For this review, take the finished solid that the model builds, in its own axes (mm). Face numbers are marked on the shaded views. Round coordinates to 2 decimals unless told otherwise and drop trailing zeros. Write each loop counter-clockwise with the first axis right and the second up, starting at its lowest first coordinate (ties: lowest second). Pieces come first, ordered by that corner, then holes. Notation, with made-up numbers: (70, 38.25) - (79, 38.25) arc R18 ccw to (79, 42.25) - close; hole circle Ø10 at (-34, 38). An arc over 180 degrees is marked (long way). One line per item, written item: value. Start each with the question number.
Q1. Add section C-C on z = 38. Write out the cut boundary in (x, y) (1 decimal), and give its area (3 significant figures).
Q2. Clearance check with flat-ended pins moving along their axes: pin 1 Ø5 at (y, z) = (1.5, 21) entering from +X; pin 2 Ø3 at (y, z) = (-4.5, 26) entering from +X; pin 3 Ø5 at (x, z) = (6, 38) entering from +Y; pin 4 Ø1.5 at (y, z) = (2, 42) entering from -X. State where each tip first meets the part, or that it passes through.
Q3. Add section A-A on y = 0. Write out the cut boundary in (x, z).
Q4. For probe 1 along Y at (x, z) = (0, 12); probe 2 along Y at (x, z) = (3.5, 27), list the stretches that pass through material, from the lowest coordinate up.
Q5. Mouldability with a two-part tool opening along Y and no side actions: class the marked faces 1, 2 and 3 as +Y half, -Y half, draft (parallel to the pull), parting line (faces both ways), or undercut.
Q6. Add section B-B on x = 0. Write out the cut boundary in (y, z).
Q7. Add section D-D on y = 6.5. Write out the cut boundary in (x, z), and give its area (3 significant figures).
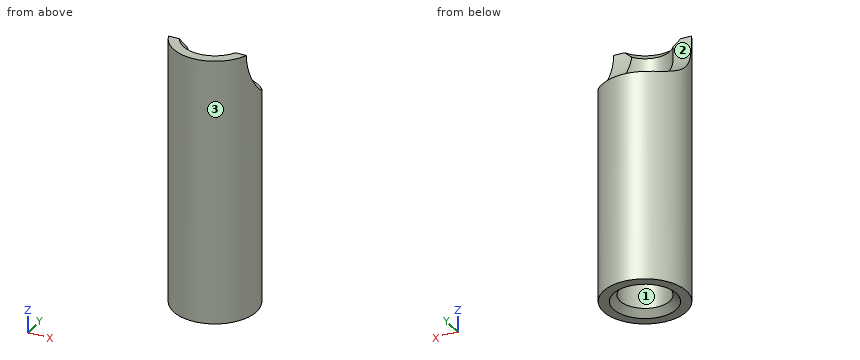
```python
from build123d import *

# Parameters (mm, degrees)
SKETCH2_R             = 7.9375
SKETCH2_R_2           = 4.7625
TUBE_DEPTH            = 50.8
CHAMFER1_SIZE         = 1.27
CURVED_CUT_DEPTH      = 53.025453506
CURVED_CUT_DEPTH_BACK = 53.025453506
SKETCH3_R             = 10.727398282


with BuildPart() as part:
    # Sketch2 → tube (new body)
    with BuildSketch(Plane.XY):
        Circle(SKETCH2_R)
        Circle(SKETCH2_R_2, mode=Mode.SUBTRACT)
    extrude(amount=TUBE_DEPTH)

    # Chamfer1
    chamfer1_edges = [part.edges().sort_by_distance(p)[0] for p in [
        (-4.7625, 0, 0),
        (-4.7625, 0, 50.8),
    ]]
    chamfer(chamfer1_edges, length=CHAMFER1_SIZE)

    # Sketch3 → curved_cut (cut, two sides: drawn at the far end of the back side and taken through both)
    with BuildSketch(Plane(origin=(0, 0, 0), x_dir=(0, 0, -1), z_dir=(1, 0, 0)).offset(-CURVED_CUT_DEPTH_BACK)):
        with Locations((-50.8, 7.9375)):
            Circle(SKETCH3_R)
    extrude(amount=CURVED_CUT_DEPTH + CURVED_CUT_DEPTH_BACK, mode=Mode.SUBTRACT)


solid = part.part
```
Result set:
1. outline: circle Ø15.9 at (0, 0); hole circle Ø9.5 at (0, 0)
1. area: 127 mm^2
2. pin 1: stops at x = 7.94
2. pin 2: stops at x = 7.35
2. pin 3: stops at y = 7.12
2. pin 4: stops at x = -7.84
3. outline: (-7.94, 0) - (-6.03, 0) - (-4.76, 1.27) - (-4.76, 43.58) - (-7.94, 43.58) - close; (4.76, 1.27) - (6.03, 0) - (7.94, 0) - (7.94, 43.58) - (4.76, 43.58) - close
4. probe 1: y = -7.94 to -4.76, 4.76 to 7.94
4. probe 2: y = -7.12 to -3.23, 3.23 to 7.12
5. face 1: undercut
5. face 2: +Y half
5. face 3: parting line
6. outline: (-7.94, 0) - (-6.03, 0) - (-4.76, 1.27) - (-4.76, 49.53) - (-6.03, 50.8) - (-7.94, 50.8) - close; (4.76, 1.27) - (6.03, 0) - (7.94, 0) - (7.94, 40.07) arc R10.73 cw to (4.76, 40.55) - close
7. outline: (-4.56, 0) - (4.56, 0) - (4.56, 40.17) - (-4.56, 40.17) - close
7. area: 366 mm^2
